from build123d import *

# Parameters (mm, degrees)
BOX007_W          = 10
BOX007_H          = 10
BOX007_DEPTH      = 10
BOX008_W          = 10
BOX008_H          = 10
BOX008_DEPTH      = 10
CYLINDER003_R     = 1.6
CYLINDER003_DEPTH = 30
CYLINDER002_R     = 1.6
CYLINDER002_DEPTH = 30
CYLINDER001_R     = 2
CYLINDER001_DEPTH = 7
CYLINDER_R        = 2
CYLINDER_DEPTH    = 7
BOX_W             = 28
BOX_H             = 30
BOX_DEPTH         = 20
FILLET_R          = 2
CYLINDER005_R     = 3.15
CYLINDER005_DEPTH = 30
CYLINDER004_R     = 6
CYLINDER004_DEPTH = 8
CYLINDER007_R     = 6
CYLINDER007_DEPTH = 21
CYLINDER006_R     = 3.15
CYLINDER006_DEPTH = 30
BOX003_W          = 75
BOX003_H          = 27
BOX003_DEPTH      = 24
CHAMFER002_SIZE2  = 26
CHAMFER002_SIZE   = 17.5
BOX004_W          = 11
BOX004_H          = 27
BOX004_DEPTH      = 14
CHAMFER_SIZE      = 10
BOX005_W          = 75
BOX005_H          = 7.8
BOX005_DEPTH      = 2
CHAMFER003_SIZE   = 1
CHAMFER004_SIZE   = 1


with BuildPart() as cube007:
    # Box007 → Box007 (new body)
    with BuildSketch(Plane(origin=(-20, 10, 26), x_dir=(1, 0, 0), z_dir=(0, 0, 1))):
        with Locations((5, 5)):
            Rectangle(BOX007_W, BOX007_H)
    extrude(amount=BOX007_DEPTH)


with BuildPart() as fusion002011:
    # Box008 → Box008 (new body)
    with BuildSketch(Plane(origin=(38, 10, 26), x_dir=(1, 0, 0), z_dir=(0, 0, 1))):
        with Locations((5, 5)):
            Rectangle(BOX008_W, BOX008_H)
    extrude(amount=BOX008_DEPTH)

    # Fusion002011: union Cube007
    add(cube007.part)


with BuildPart() as cylinder003:
    # Cylinder003 → Cylinder003 (new body)
    with BuildSketch(Plane(origin=(-20, 0, 17), x_dir=(1, 0, 0), z_dir=(0, 1, 0))):
        Circle(CYLINDER003_R)
    extrude(amount=CYLINDER003_DEPTH)


with BuildPart() as cylinder002:
    # Cylinder002 → Cylinder002 (new body)
    with BuildSketch(Plane(origin=(20, 0, 17), x_dir=(1, 0, 0), z_dir=(0, 1, 0))):
        Circle(CYLINDER002_R)
    extrude(amount=CYLINDER002_DEPTH)


with BuildPart() as cylinder001:
    # Cylinder001 → Cylinder001 (new body)
    with BuildSketch(Plane(origin=(20, 0, 17), x_dir=(1, 0, 0), z_dir=(0, 1, 0))):
        Circle(CYLINDER001_R)
    extrude(amount=CYLINDER001_DEPTH)


with BuildPart() as cylinder:
    # Cylinder → Cylinder (new body)
    with BuildSketch(Plane(origin=(-20, 0, 17), x_dir=(1, 0, 0), z_dir=(0, 1, 0))):
        Circle(CYLINDER_R)
    extrude(amount=CYLINDER_DEPTH)


with BuildPart() as plug_slot:
    # Box → Box (new body)
    with BuildSketch(Plane(origin=(-14, 0, 7), x_dir=(1, 0, 0), z_dir=(0, 0, 1))):
        with Locations((14, 15)):
            Rectangle(BOX_W, BOX_H)
    extrude(amount=BOX_DEPTH)

    # Fillet
    fillet_edges = [plug_slot.edges().sort_by_distance(p)[0] for p in [
        (-14, 15, 27),
        (-14, 15, 7),
        (14, 15, 27),
        (14, 15, 7),
    ]]
    fillet(fillet_edges, radius=FILLET_R)

    # Fusion: union Cylinder003, Cylinder002, Cylinder001, Cylinder
    add(cylinder003.part)
    add(cylinder002.part)
    add(cylinder001.part)
    add(cylinder.part)


with BuildPart() as plug_slot_1:
    # Fusion placement: moved
    add(plug_slot.part.moved(Location((13, 0, -3))))


with BuildPart() as cylinder005:
    # Cylinder005 → Cylinder005 (new body)
    with BuildSketch(Plane(origin=(0, 15, 0), x_dir=(1, 0, 0), z_dir=(0, 0, 1))):
        Circle(CYLINDER005_R)
    extrude(amount=CYLINDER005_DEPTH)


with BuildPart() as fusion002009:
    # Cylinder004 → Cylinder004 (new body)
    with BuildSketch(Plane(origin=(0, 15, 0), x_dir=(1, 0, 0), z_dir=(0, 0, 1))):
        Circle(CYLINDER004_R)
    extrude(amount=CYLINDER004_DEPTH)

    # Fusion002009: union Cylinder005
    add(cylinder005.part)


with BuildPart() as fusion002009_1:
    # Fusion002009 placement: moved
    add(fusion002009.part.moved(Location((-15, 0, 0))))


with BuildPart() as cylinder007:
    # Cylinder007 → Cylinder007 (new body)
    with BuildSketch(Plane(origin=(43, 15, 0), x_dir=(1, 0, 0), z_dir=(0, 0, 1))):
        Circle(CYLINDER007_R)
    extrude(amount=CYLINDER007_DEPTH)


with BuildPart() as fusion002010:
    # Cylinder006 → Cylinder006 (new body)
    with BuildSketch(Plane(origin=(43, 15, 0), x_dir=(1, 0, 0), z_dir=(0, 0, 1))):
        Circle(CYLINDER006_R)
    extrude(amount=CYLINDER006_DEPTH)

    # Fusion002005: union Cylinder007
    add(cylinder007.part)

    # Fusion002010: union Fusion002009
    add(fusion002009_1.part)


with BuildPart() as chamfer002:
    # Box003 → Box003 (new body)
    with BuildSketch(Plane(origin=(-23, 0, 2), x_dir=(1, 0, 0), z_dir=(0, 0, 1))):
        with Locations((37.5, 13.5)):
            Rectangle(BOX003_W, BOX003_H)
    extrude(amount=BOX003_DEPTH)

    # Chamfer002
    chamfer002_edges = [chamfer002.edges().sort_by_distance(p)[0] for p in [
        (52, 13.5, 2),
    ]]
    chamfer002_side = chamfer002.faces().sort_by_distance((52, 13.5, 14))[0]
    chamfer(chamfer002_edges, length=CHAMFER002_SIZE, length2=CHAMFER002_SIZE2, reference=chamfer002_side)


with BuildPart() as chamfer_body:
    # Box004 → Box004 (new body)
    with BuildSketch(Plane(origin=(-33, 0, 2), x_dir=(1, 0, 0), z_dir=(0, 0, 1))):
        with Locations((5.5, 13.5)):
            Rectangle(BOX004_W, BOX004_H)
    extrude(amount=BOX004_DEPTH)

    # Chamfer
    chamfer_edges = [chamfer_body.edges().sort_by_distance(p)[0] for p in [
        (-33, 13.5, 16),
    ]]
    chamfer(chamfer_edges, length=CHAMFER_SIZE)


with BuildPart() as cut008004003004014002002008002001:
    # Box005 → Box005 (new body)
    with BuildSketch(Plane(origin=(-23, 11.1, 25), x_dir=(1, 0, 0), z_dir=(0, 0, 1))):
        with Locations((37.5, 3.9)):
            Rectangle(BOX005_W, BOX005_H)
    extrude(amount=BOX005_DEPTH)

    # Chamfer003
    chamfer003_edges = [cut008004003004014002002008002001.edges().sort_by_distance(p)[0] for p in [
        (14.5, 18.9, 27),
    ]]
    chamfer(chamfer003_edges, length=CHAMFER003_SIZE)

    # Fusion002008: union Chamfer002, Chamfer body
    add(chamfer002.part)
    add(chamfer_body.part)

    # Cut: cut Fusion002010
    add(fusion002010.part, mode=Mode.SUBTRACT)

    # Cut008004003004014002002008: cut plug-slot
    add(plug_slot_1.part, mode=Mode.SUBTRACT)

    # Chamfer004
    chamfer004_edges = [cut008004003004014002002008002001.edges().sort_by_distance(p)[0] for p in [
        (39, 0, 10.75),
        (39, 27, 10.75),
        (-23, 27, 21),
        (-23, 0, 21),
        (-28, 0, 11),
        (-28, 27, 11),
        (-33, 0, 4),
        (-33, 13.5, 2),
        (-33, 27, 4),
        (52, 0, 22.75),
        (52, 27, 22.75),
        (-3.5, 27, 2),
        (-3.5, 0, 2),
    ]]
    chamfer(chamfer004_edges, length=CHAMFER004_SIZE)

    # Cut008004003004014002002008002: cut Fusion002011
    add(fusion002011.part, mode=Mode.SUBTRACT)


solid = cut008004003004014002002008002001.part
Input: part model. Units: mm. Frame: model coordinates. A direction names the side the tool comes from. Give positions to 0.01 mm unless a question says otherwise; leave off trailing zeros. Write each loop counter-clockwise with the first axis right and the second up, starting at its lowest first coordinate (ties: lowest second). Pieces come first, ordered by that corner, then holes. Notation, with made-up numbers: (-16, 37) -> (3, 37) arc R22 ccw to (3, 59) -> close; hole circle Ø6 at (13, 41.25). An arc over 180 degrees is marked (long way). Use one line per item in the form item = value. Start each with the question number.
1) Section query D-D on y = 13. Count the separate pieces of the cut face and the enclosed holes in it, then the cut area to 3 significant figures.
2) Pin query (flat end, axial travel): pin 1 (12 mm diameter, centred on x = 28.5, y = 6.5, fed in from -Z); pin 2 (3.5 mm diameter, centred on x = -13.5, y = 14.5, fed in from -Z); pin 3 (10 mm diameter, centred on y = 15.5, z = 11, fed in from +X); pin 4 (1.1 mm diameter, centred on y = 13.5, z = 26.5, fed in from -X). Return the tip coordinate at first contact, or that it passes through.
3) Section query B-B on z = 4.75. Return the cut outline in (x, y), then the cut area to 3 significant figures.
4) Section query C-C on x = -15. Return the cut outline in (y, z), then the cut area to 3 significant figures.
5) Section query A-A on x = 19. Return the cut outline in (y, z).
6) Ray query, probe 1 along X at (y, z) = (15, 25.05); probe 2 along Z at (x, y) = (14, 14.75); probe 3 along Y at (x, z) = (-15, 4.9). Return the intervals inside material, ascending. Write a range as from..to.
7) Set-up query: faces 4 (the flat face through (-28, 13, 11)), 5 (the cylindrical face through (-9.277, 16.802, 4.958)), 6 (the cylindrical face through (-8.474, 3.451, 12.648)), 7 (the flat face through (-27.567, 26.507, 10.716)), 8 (the cylindrical face through (26.43, 13.69, 4.6)). Return all of +Z, -Z, +X, -X, +Y, -Y with unobstructed straight access to the full face (end or side cutting, diameter ignored); none if empty.
8) Draft query along X for faces 1 (the flat face through (38.91, 0.51, 11.28)), 2 (the flat face through (50, 15, 27)), 3 (the cylindrical face through (-8.18, 16.86, 12.92)). Return one class per face: pulls with the +X half, pulls with the -X half, needs draft (parallel to the pull), parting line crosses it, or undercut.
Outcome:
q1.separate_pieces = 3
q1.enclosed_holes = 3
q1.area = 879 mm^2
q2.pin_1 = 2
q2.pin_2 = 8
q2.pin_3 = 40.48
q2.pin_4 = -23
q3.outline = (-33, 1) -> (-32, 0) -> (-0.56, 0) -> (-0.56, 27) -> (-32, 27) -> (-33, 26) -> close; (26.56, 0) -> (28.29, 0) -> (30.09, 1) -> (30.09, 26) -> (28.29, 27) -> (26.56, 27) -> close; hole circle Ø12 at (-15, 15)
q3.area = 855 mm^2
q4.outline = (0, 3) -> (1, 2) -> (9, 2) -> (9, 8) -> (11.85, 8) -> (11.85, 26) -> (0, 26) -> close; (18.15, 8) -> (21, 8) -> (21, 2) -> (26, 2) -> (27, 3) -> (27, 26) -> (18.15, 26) -> close
q4.area = 462 mm^2
q5.outline = (0, 3) -> (1, 2) -> (26, 2) -> (27, 3) -> (27, 4) -> (0, 4) -> close; (0, 24) -> (27, 24) -> (27, 26) -> (18.9, 26) -> (17.9, 27) -> (11.1, 27) -> (11.1, 26) -> (0, 26) -> close
q6.probe_1 = -23..-18.15, -11.85..39.85, 46.15..52
q6.probe_2 = 2..4, 24..27
q6.probe_3 = 0..9, 21..27
q7.face_4 = +Z, -X, +Y, -Y
q7.face_5 = -Z
q7.face_6 = -Y
q7.face_7 = +Z, -X, +Y
q7.face_8 = +Y, -Y
q8.face_1 = pulls with the +X half
q8.face_2 = needs draft
q8.face_3 = undercut
